from build123d import *

# Parameters (mm, degrees)
SKETCH1_R           = 4.000000001
SKETCH1_R_2         = 3.175
SKETCH1_R_3         = 9.525
BOSS_EXTRUDE1_DEPTH = 4.7625
FILLET1_R           = 6.35
CUT_EXTRUDE4_DEPTH  = 1.27


with BuildPart() as part:
    # Sketch1 → Boss-Extrude1 (new body)
    with BuildSketch(Plane(origin=(0, 0, 0), x_dir=(0, 0, -1), z_dir=(1, 0, 0))):
        with BuildLine():
            Line((7.857724106, 7.857724106), (-21.748484988, 37.4639332))
            Line((-21.748484988, 37.4639332), (-81.276178769, 37.4639332))
            Line((-81.276178769, 37.4639332), (-81.276178769, -11.1125))
            Line((-81.276178769, -11.1125), (0, -11.1125))
            ThreePointArc((0, -11.1125), (10.266611305, -4.252569642), (7.857724106, 7.857724106))
        make_face()
        with Locations(Location((0, 0, 0), (0, 0, 180))):
            Circle(SKETCH1_R, mode=Mode.SUBTRACT)
        with Locations(Location((-68.576178769, 24.7639332, 0), (0, 0, 180))):
            Circle(SKETCH1_R_2, mode=Mode.SUBTRACT)
        with Locations(Location((-45.399745569, 24.7639332, 0), (0, 0, 180))):
            Circle(SKETCH1_R_2, mode=Mode.SUBTRACT)
        with Locations(Location((-45.399745569, 1.5875, 0), (0, 0, 180))):
            Circle(SKETCH1_R_2, mode=Mode.SUBTRACT)
        with Locations(Location((-68.576178769, 1.5875, 0), (0, 0, 180))):
            Circle(SKETCH1_R_2, mode=Mode.SUBTRACT)
        with Locations(Location((-56.987962169, 13.1757166, 0), (0, 0, 180))):
            Circle(SKETCH1_R_3, mode=Mode.SUBTRACT)
    extrude(amount=BOSS_EXTRUDE1_DEPTH)

    # Fillet1
    fillet1_edges = [part.edges().sort_by_distance(p)[0] for p in [
        (2.38125, -11.1125, 81.276178769),
        (2.38125, 37.4639332, 81.276178769),
        (2.38125, 37.4639332, 21.748484988),
    ]]
    fillet(fillet1_edges, radius=FILLET1_R)

    # Sketch5 → Cut-Extrude4 (cut)
    with BuildSketch(Plane.ZY):
        with BuildLine():
            Line((35.620745569, 24.7639332), (35.620745569, 1.5875))
            ThreePointArc((35.620745569, 1.5875), (38.484948356, -5.327297213), (45.399745569, -8.1915))
            Line((45.399745569, -8.1915), (68.576178769, -8.1915))
            ThreePointArc((68.576178769, -8.1915), (75.490975982, -5.327297213), (78.355178769, 1.5875))
            Line((78.355178769, 1.5875), (78.355178769, 24.7639332))
            ThreePointArc((78.355178769, 24.7639332), (75.490975982, 31.678730413), (68.576178769, 34.5429332))
            Line((68.576178769, 34.5429332), (45.399745569, 34.5429332))
            ThreePointArc((45.399745569, 34.5429332), (38.484948356, 31.678730413), (35.620745569, 24.7639332))
        make_face()
    extrude(amount=-CUT_EXTRUDE4_DEPTH, mode=Mode.SUBTRACT)


solid = part.part
Work out the finished part from the listing and answer in its coordinate system (mm). A direction names the side the tool comes from. Give positions to 0.01 mm unless a question says otherwise; leave off trailing zeros. Order: outer loops, then holes, each group sorted by start corner. A loop starts at its lowest first (then second) coordinate and runs counter-clockwise, first axis right, second up. Notation, with made-up numbers: (43, 72.5) - (81, 72.5) arc R21 cw to (81, 93.5) - close; hole circle Ø2 at (16.5, 42). An arc over 180 degrees is marked (long way). Answer as CSV lines item,"result". Start each with the question number.
Q1. The part is cut by section B-B (y = 0). Write down the section's boundary in (x, z), then the cut area to 3 significant figures.
Q2. The part is cut by section A-A (x = 3.35). Give the number of separate pieces and of enclosed holes in the cut face, then the cut area to 3 significant figures.
Q3. Given pin 1 Ø8.5 at (y, z) = (1.59, 68.58) entering from -X; pin 2 Ø1 at (x, y) = (0.5, 19) entering from -Z, each flat-ended and moving along its own axis, determine where each tip first touches the part or whether it passes through.
Q4. The mould has two halves that part along Z. Classify faces 1 (the face through (2, 13, 81.276)), 2 (the face through (2.99, 18.97, 49.43)), 3 (the face through (2.992, 1.448, 65.404)), 4 (the face through (2, 37.464, 49)): +Z half, -Z half, draft (parallel to the pull), parting line (faces both ways), or undercut.
Q5. For faces 5 (the face through (0.626, -5.403, 75.415)), 6 (the face through (2.35, -2.7, -2.95)), determine the directions among +Z, -Z, +X, -X, +Y, -Y from which every point of the face is accessible in a straight line to the end or side of a thin tool.
Q6. Find the intervals of material crossed by L1, parallel to Y at x = 1.1, z = 51; L2, parallel to Z at x = 2.8, y = 0.5; L3, parallel to Y at x = 1.5, z = 68, in increasing order. Write a range as [from, to].
Q7. The part is cut by section C-C (y = 17). Write down the section's boundary in (x, z).
Check result:
1,outline,"(0, -11.11) - (4.76, -11.11) - (4.76, -4) - (0, -4) - close; (0, 4) - (4.76, 4) - (4.76, 42.65) - (1.27, 42.65) - (1.27, 35.75) - (0, 35.75) - close; (0, 78.23) - (1.27, 78.23) - (1.27, 71.33) - (4.76, 71.33) - (4.76, 81.28) - (0, 81.28) - close; (1.27, 48.15) - (4.76, 48.15) - (4.76, 65.83) - (1.27, 65.83) - close"
1,area,"310 mm²"
2,separate pieces,"1"
2,enclosed holes,"6"
2,area,"3,440 mm²"
3,pin 1,"stops at x = 1.27"
3,pin 2,"stops at z = 2.78"
4,face 1,"+Z half"
4,face 2,"undercut"
4,face 3,"undercut"
4,face 4,"draft"
5,face 5,"-X"
5,face 6,"+X, -X"
6,L1,"y = [-11.11, -8.19], [34.54, 37.46]"
6,L2,"z = [-11.1, -3.97], [3.97, 42.42], [48.38, 65.59], [71.56, 81.28]"
6,L3,"y = [-11.11, -1.53], [4.71, 21.64], [27.89, 37.46]"
7,outline,"(0, 1.28) - (4.76, 1.28) - (4.76, 48.26) - (1.27, 48.26) - (1.27, 35.62) - (0, 35.62) - close; (0, 78.36) - (1.27, 78.36) - (1.27, 65.71) - (4.76, 65.71) - (4.76, 81.28) - (0, 81.28) - close"
